Can you work these out from the model? Positions are in its coordinate system, mm. Face numbers are marked on the shaded views. Coordinates: 2 decimals unless noted, no trailing zeros. Loops run counter-clockwise (first coordinate to the right, second up) from the corner with the lowest first, then second, coordinate; pieces in that order, holes last.
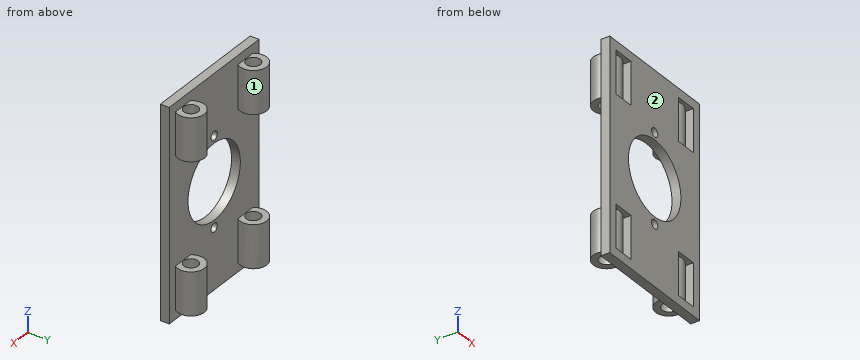
Autodesk Inventor part; units mm, degrees
ref_plane "YZ Plane" through (0, 0, 0) normal (1, 0, 0) x (0, 1, 0)
ref_plane "XZ Plane" through (0, 0, 0) normal (0, 1, 0) x (-1, 0, 0)
ref_plane "XY Plane" through (0, 0, 0) normal (0, 0, 1) x (1, 0, 0)
sketch "Sketch1" plane through (0, 0, 0) normal (0, 1, 0) x (-1, 0, 0)
  circle A0 centre (0, 0) radius 21
  circle A1 centre (0, 25) radius 2.5
  circle A2 centre (0, -25) radius 2.5
  line L0 (-31, 54) -> (-19, 54)
  line L1 (-19, 54) -> (-19, 30)
  line L2 (-19, 30) -> (-31, 30)
  line L3 (-31, 30) -> (-31, 54)
  line L4 (19, 54) -> (31, 54)
  line L5 (31, 54) -> (31, 30)
  line L6 (31, 30) -> (19, 30)
  line L7 (19, 30) -> (19, 54)
  line L8 (-31, -30) -> (-19, -30)
  line L9 (-19, -30) -> (-19, -54)
  line L10 (-19, -54) -> (-31, -54)
  line L11 (-31, -54) -> (-31, -30)
  line L12 (19, -30) -> (31, -30)
  line L13 (31, -30) -> (31, -54)
  line L14 (31, -54) -> (19, -54)
  line L15 (19, -54) -> (19, -30)
  line L16 (-36, 59) -> (36, 59)
  line L17 (36, 59) -> (36, -59)
  line L18 (36, -59) -> (-36, -59)
  line L19 (-36, -59) -> (-36, 59)
  dimension "d2" = 5
  dimension "d4" = 5
  dimension "d9" = 12
  dimension "d10" = 24
  dimension "d11" = 12
  dimension "d12" = 24
  dimension "d13" = 12
  dimension "d14" = 24
  dimension "d15" = 12
  dimension "d16" = 24
extrude "Extrusion1" add sketch "Sketch1" along normal blind 5
sketch "Sketch2" plane through (19, 0, 30) normal (0, 0, 1) x (1, 0, 0)
  line L0 (0, 5) -> (12, 5)
  line L1 (0, 0) -> (0, 5)
  line L2 (6, 5) -> (6, 9.5)
  circle A0 centre (6, 9.5) radius 7.5
  circle A1 centre (6, 9.5) radius 4
  point P0 (-19, 0)
  dimension "d23" = 4.5
  dimension "d24" = 15
  dimension "d25" = 8
extrude "Extrusion2" add sketch "Sketch2" along normal blind 24
sketch "Sketch3" plane through (-31, 0, 30) normal (0, 0, 1) x (1, 0, 0)
  line L0 (0, 5) -> (12, 5)
  line L1 (0, 0) -> (0, 5)
  line L2 (6, 5) -> (6, 9.5)
  circle A0 centre (6, 9.5) radius 7.5
  circle A1 centre (6, 9.5) radius 4
  point P0 (31, 0)
  dimension "d28" = 4.5
  dimension "d29" = 15
  dimension "d30" = 8
extrude "Extrusion3" add sketch "Sketch3" along normal blind 24
sketch "Sketch4" plane through (-19, 0, -30) normal (0, 0, -1) x (-1, 0, 0)
  line L0 (0, 5) -> (12, 5)
  line L1 (0, 0) -> (0, 5)
  line L2 (6, 5) -> (6, 9.5)
  circle A0 centre (6, 9.5) radius 7.5
  circle A1 centre (6, 9.5) radius 4
  point P0 (-19, 0)
  dimension "d33" = 4.5
  dimension "d34" = 15
  dimension "d35" = 8
extrude "Extrusion4" add sketch "Sketch4" along normal blind 24
sketch "Sketch5" plane through (31, 0, -30) normal (0, 0, -1) x (-1, 0, 0)
  line L0 (0, 5) -> (12, 5)
  line L1 (0, 0) -> (0, 5)
  line L2 (6, 5) -> (6, 9.5)
  circle A0 centre (6, 9.5) radius 7.5
  circle A1 centre (6, 9.5) radius 4
  point P0 (31, 0)
  dimension "d38" = 4.5
  dimension "d39" = 15
  dimension "d40" = 8
extrude "Extrusion5" add sketch "Sketch5" along normal blind 24
properties part number "X_Carriage_V1" material "Ash"
Item 1: We'd pull the mould along Y, two halves only. Please class the marked faces 1 and 2: +Y half, -Y half, draft (parallel to the pull), parting line (faces both ways), or undercut.
Results are:
face 1: undercut
face 2: -Y half
Item 2: Suppose I cut it at D-D, the plane y = 11.75. Count the separate pieces of the cut face and the enclosed holes in it, plus the area to 3 significant figures.
Results are:
separate pieces: 8
enclosed holes: 0
area: 739 mm2
Item 3: I'm going to push flat-ended pins straight in: P1, Ø4.5, axis at x = 0, z = -25, coming from the -Y side; P2, Ø1.5, axis at x = -21, z = 40.5, coming from the -Y side; P3, Ø5, axis at y = 12.5, z = -33, coming from the -X side. Where does each tip first touch, or does it pass through?
Results are:
P1: passes through
P2: stops at y = 2.74
P3: stops at x = -32.48
Item 4: Suppose I cut it at B-B, the plane x = 0. Please give me the cut outline in (y, z), plus the area to 3 significant figures.
Results are:
outline: (0, -59) - (5, -59) - (5, -27.5) - (0, -27.5) - close; (0, -22.5) - (5, -22.5) - (5, -21) - (0, -21) - close; (0, 21) - (5, 21) - (5, 22.5) - (0, 22.5) - close; (0, 27.5) - (5, 27.5) - (5, 59) - (0, 59) - close
area: 330 mm2
Item 5: Suppose I cut it at C-C, the plane z = -25. Please give me the cut outline in (x, y), plus the area to 3 significant figures.
Results are:
outline: (-36, 0) - (-2.5, 0) - (-2.5, 5) - (-36, 5) - close; (2.5, 0) - (36, 0) - (36, 5) - (2.5, 5) - close
area: 335 mm2
Item 6: I need wall thicknesses on line 1 along Z through (x, y) = (0, 3.6); line 2 along Z through (x, y) = (26.5, 1); line 3 along Z through (x, y) = (-22, 12.5). Which ranges of each line are inside material? Lowest first, please.
Results are:
line 1: z = -59 to -27.5, -22.5 to -21, 21 to 22.5, 27.5 to 59
line 2: z = -59 to -54, -30 to 30, 54 to 59
line 3: z = -54 to -30, 30 to 54
